Build history of the part. All positions in model axes, mm. Face numbers are marked on the shaded views. Round coordinates to 2 decimals unless told otherwise and drop trailing zeros. Loops run counter-clockwise (first coordinate to the right, second up) from the corner with the lowest first, then second, coordinate; pieces in that order, holes last. Notation, with made-up numbers: (12.25, 58.25) -> (61.25, 58.25) arc R21 ccw to (61.25, 78.25) -> close; hole circle Ø4 at (-2, 18.25). An arc over 180 degrees is marked (long way). Put each result on its own line as item: value. Start each with the question number.
Item 1: Drill centre lines: probe 1 along Y at (x, z) = (60, 26.3); probe 2 along X at (y, z) = (19.5, 25.75); probe 3 along X at (y, z) = (9.5, 23). Where is each one in solid material? Low to high. Write a range as [from, to].
Item 2: Cut at C-C, the plane x = 115. List the corners of the cut face in (y, z).
Item 3: Pull direction Y, two halves, no side cores. Call the marked faces 1, 2, 3 and 4: +Y half, -Y half, draft (parallel to the pull), parting line (faces both ways), or undercut.
Item 4: Cut at A-A, the plane y = 5. List the corners of the cut face in (x, z).
Item 5: Cut at D-D, the plane z = 28.5. Count the separate pieces of the cut face and the enclosed holes in it, plus the area to 3 significant figures.
Item 6: Flat gauge pin, fed straight in: pin 1 Ø0.8 at (x, z) = (61, 23.5) entering from +Y. Where does the tip first touch, or does it go through?
Item 7: Cut at B-B, the plane x = 5. List the corners of the cut face in (y, z).
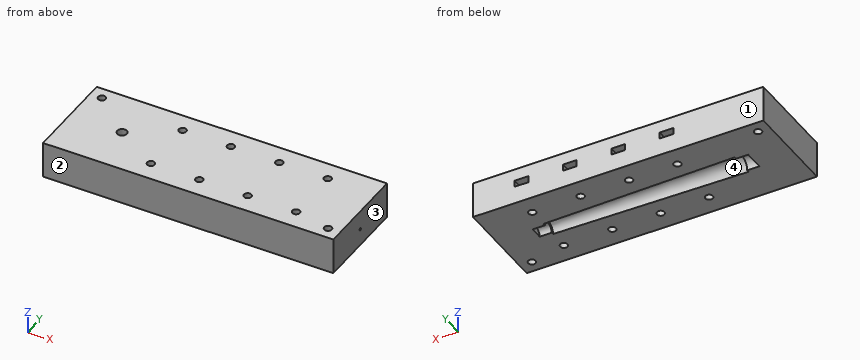
```python
from build123d import *

# Parameters (mm, degrees)
SKIZZE2_W                        = 120
SKIZZE2_H                        = 39.364160046
AUFSATZ_LINEAR_AUSTRAGEN1_DEPTH  = 30
SKIZZE24_R                       = 1.55
SCHNITT_LINEAR_AUSTRAGEN4_DEPTH  = 130.805766806
SKIZZE46_R                       = 2.85
SCHNITT_LINEAR_AUSTRAGEN15_DEPTH = 10
SCHNITT_LINEAR_START             = -5
SCHNITT_LINEAR_AUSTRAGEN25_DEPTH = 2.7
LINEARES_MUSTER1_COUNT           = 4
LINEARES_MUSTER1_PITCH           = 20
SPIEGELN2_COPY_1_SKETCH_R        = 2.85
SPIEGELN2_COPY_1_DEPTH           = 10
SPIEGELN2_COPY_2_SKETCH_R        = 2.85
SPIEGELN2_COPY_2_DEPTH           = 10
SPIEGELN2_COPY_3_SKETCH_R        = 2.85
SPIEGELN2_COPY_3_DEPTH           = 10
SPIEGELN2_START                  = -5
SPIEGELN2_COPY_4_DEPTH           = 2.7
SPIEGELN2_COPY_5_DEPTH           = 2.7
SPIEGELN2_COPY_6_DEPTH           = 2.7
SKIZZE51_R                       = 1.55
SCHNITT_LINEAR_AUSTRAGEN26_DEPTH = 130.805766806
SKIZZE75_R                       = 0.75
SCHNITT_LINEAR_AUSTRAGEN28_DEPTH = 12
SKIZZE76_R                       = 2
SCHNITT_LINEAR_AUSTRAGEN29_DEPTH = 6
SKIZZE80_R                       = 0.5
SCHNITT_LINEAR_AUSTRAGEN34_DEPTH = 21.05
SCHNITT_LINEAR_START_2           = -7.5
SKIZZE81_R                       = 0.5
SCHNITT_LINEAR_AUSTRAGEN36_DEPTH = 5
FASE1_SIZE                       = 1
ABSPALTEN3_OUTLINE_W             = 120
ABSPALTEN3_OUTLINE_H             = 39.364160046
ABSPALTEN3_OUTLINE_R             = 1.55
ABSPALTEN3_DEPTH                 = 15


# Read off the part's stored shape, not the designer's step: Abspalten3
with BuildPart() as part:
    # Skizze2 → Aufsatz-Linear austragen1 (new body)
    with BuildSketch(Plane.XY):
        with Locations((60, 19.682080023)):
            Rectangle(SKIZZE2_W, SKIZZE2_H)
    extrude(amount=AUFSATZ_LINEAR_AUSTRAGEN1_DEPTH)

    # Skizze24 → Schnitt-Linear austragen4 (cut, through all)
    with BuildSketch(Plane.XY.offset(30)):
        with Locations((40, 31.364160046)):
            Circle(SKIZZE24_R)
        with Locations((60, 31.364160046)):
            Circle(SKIZZE24_R)
        with Locations((80, 31.364160046)):
            Circle(SKIZZE24_R)
        with Locations((100, 31.364160046)):
            Circle(SKIZZE24_R)
    schnitt_linear_austragen4 = extrude(amount=-SCHNITT_LINEAR_AUSTRAGEN4_DEPTH, mode=Mode.SUBTRACT)

    # Skizze46 → Schnitt-Linear austragen15 (cut)
    with BuildSketch(Plane(origin=(0, 0, 0), x_dir=(-1, 0, 0), z_dir=(0, 0, -1))):
        with Locations((-100, 31.364160046)):
            Circle(SKIZZE46_R)
    schnitt_linear_austragen15 = extrude(amount=-SCHNITT_LINEAR_AUSTRAGEN15_DEPTH, mode=Mode.SUBTRACT)

    # Skizze50 → Schnitt-Linear austragen25 (cut)
    with BuildSketch(Plane.XY.offset(30).offset(SCHNITT_LINEAR_START)):
        Polygon((97.15, 33.009608314), (97.15, 39.364160046), (102.85, 39.364160046), (102.85, 33.009608314), (102.85, 29.718711779), (100, 28.073263512), (97.15, 29.718711779), align=None)
    schnitt_linear_austragen25 = extrude(amount=-SCHNITT_LINEAR_AUSTRAGEN25_DEPTH, mode=Mode.SUBTRACT)

    # Lineares Muster1: Schnitt-Linear austragen15, Schnitt-Linear austragen25 ×4
    with Locations(*[(-i * LINEARES_MUSTER1_PITCH, 0, 0) for i in range(1, LINEARES_MUSTER1_COUNT)]):
        add(schnitt_linear_austragen15, mode=Mode.SUBTRACT)
        add(schnitt_linear_austragen25, mode=Mode.SUBTRACT)

    # Spiegeln2: Schnitt-Linear austragen15, Schnitt-Linear austragen25 across plane
    add(schnitt_linear_austragen15.mirror(Plane.ZX.offset(19.764160046)), mode=Mode.SUBTRACT)
    add(schnitt_linear_austragen25.mirror(Plane.ZX.offset(19.764160046)), mode=Mode.SUBTRACT)

    # Spiegeln2 copy 1 sketch → Spiegeln2 copy 1 (cut)
    with BuildSketch(Plane(origin=(-20, 39.528320093, 0), x_dir=(-1, 0, 0), z_dir=(0, 0, -1))):
        with Locations((-100, -31.364160046)):
            Circle(SPIEGELN2_COPY_1_SKETCH_R)
    extrude(amount=-SPIEGELN2_COPY_1_DEPTH, mode=Mode.SUBTRACT)

    # Spiegeln2 copy 2 sketch → Spiegeln2 copy 2 (cut)
    with BuildSketch(Plane(origin=(-40, 39.528320093, 0), x_dir=(-1, 0, 0), z_dir=(0, 0, -1))):
        with Locations((-100, -31.364160046)):
            Circle(SPIEGELN2_COPY_2_SKETCH_R)
    extrude(amount=-SPIEGELN2_COPY_2_DEPTH, mode=Mode.SUBTRACT)

    # Spiegeln2 copy 3 sketch → Spiegeln2 copy 3 (cut)
    with BuildSketch(Plane(origin=(-60, 39.528320093, 0), x_dir=(-1, 0, 0), z_dir=(0, 0, -1))):
        with Locations((-100, -31.364160046)):
            Circle(SPIEGELN2_COPY_3_SKETCH_R)
    extrude(amount=-SPIEGELN2_COPY_3_DEPTH, mode=Mode.SUBTRACT)

    # Spiegeln2 copy 4 sketch → Spiegeln2 copy 4 (cut)
    with BuildSketch(Plane(origin=(-20, 39.528320093, 30), x_dir=(1, 0, 0), z_dir=(0, 0, 1)).offset(SPIEGELN2_START)):
        Polygon((97.15, -33.009608314), (97.15, -39.364160046), (102.85, -39.364160046), (102.85, -33.009608314), (102.85, -29.718711779), (100, -28.073263512), (97.15, -29.718711779), align=None)
    extrude(amount=-SPIEGELN2_COPY_4_DEPTH, mode=Mode.SUBTRACT)

    # Spiegeln2 copy 5 sketch → Spiegeln2 copy 5 (cut)
    with BuildSketch(Plane(origin=(-40, 39.528320093, 30), x_dir=(1, 0, 0), z_dir=(0, 0, 1)).offset(SPIEGELN2_START)):
        Polygon((97.15, -33.009608314), (97.15, -39.364160046), (102.85, -39.364160046), (102.85, -33.009608314), (102.85, -29.718711779), (100, -28.073263512), (97.15, -29.718711779), align=None)
    extrude(amount=-SPIEGELN2_COPY_5_DEPTH, mode=Mode.SUBTRACT)

    # Spiegeln2 copy 6 sketch → Spiegeln2 copy 6 (cut)
    with BuildSketch(Plane(origin=(-60, 39.528320093, 30), x_dir=(1, 0, 0), z_dir=(0, 0, 1)).offset(SPIEGELN2_START)):
        Polygon((97.15, -33.009608314), (97.15, -39.364160046), (102.85, -39.364160046), (102.85, -33.009608314), (102.85, -29.718711779), (100, -28.073263512), (97.15, -29.718711779), align=None)
    extrude(amount=-SPIEGELN2_COPY_6_DEPTH, mode=Mode.SUBTRACT)

    # Spiegeln3: Schnitt-Linear austragen4 across plane
    add(schnitt_linear_austragen4.mirror(Plane.ZX.offset(19.764160046)), mode=Mode.SUBTRACT)

    # Skizze51 → Schnitt-Linear austragen26 (cut, through all)
    with BuildSketch(Plane.XY.offset(30)):
        with Locations((5, 34.364160046)):
            Circle(SKIZZE51_R)
        with Locations((115, 5)):
            Circle(SKIZZE51_R)
    extrude(amount=-SCHNITT_LINEAR_AUSTRAGEN26_DEPTH, mode=Mode.SUBTRACT)

    # Skizze73 → Schnitt-Rotation5 (revolve, cut)
    with BuildSketch(Plane.XY.offset(15)):
        Polygon((15, 19.764160046), (15, 23.814160046), (20, 23.814160046), (20, 24.814160046), (100, 23.232080023), (100, 22.232080023), (105, 22.232080023), (105, 19.682080023), align=None)
    revolve(axis=Axis((105, 19.682080023, 15), (-0.9999995841280241, 0.0009119998787298228, 0)), mode=Mode.SUBTRACT)

    # Skizze75 → Schnitt-Linear austragen28 (cut)
    with BuildSketch(Plane.XY.offset(30)):
        with Locations((21.598259807, 19.682080023)):
            Circle(SKIZZE75_R)
    extrude(amount=-SCHNITT_LINEAR_AUSTRAGEN28_DEPTH, mode=Mode.SUBTRACT)

    # Skizze76 → Schnitt-Linear austragen29 (cut)
    with BuildSketch(Plane.XY.offset(30)):
        with Locations((21.598259807, 19.682080023)):
            Circle(SKIZZE76_R)
    extrude(amount=-SCHNITT_LINEAR_AUSTRAGEN29_DEPTH, mode=Mode.SUBTRACT)

    # Skizze80 → Schnitt-Linear austragen34 (cut)
    with BuildSketch(Plane(origin=(120, 0, 0), x_dir=(0, 0, -1), z_dir=(1, 0, 0))):
        with Locations((-22.000416524, 19.763714623)):
            Circle(SKIZZE80_R)
    schnitt_linear_austragen34 = extrude(amount=-SCHNITT_LINEAR_AUSTRAGEN34_DEPTH, mode=Mode.SUBTRACT)

    # Skizze81 → Schnitt-Linear austragen36 (cut)
    with BuildSketch(Plane.XY.offset(30).offset(SCHNITT_LINEAR_START_2)):
        with Locations(Location((99, 19.682080023, 0), (0, 0, 7.034090001))):
            Circle(SKIZZE81_R)
    schnitt_linear_austragen36 = extrude(amount=-SCHNITT_LINEAR_AUSTRAGEN36_DEPTH, mode=Mode.SUBTRACT)

    # Spiegeln4: Schnitt-Linear austragen34, Schnitt-Linear austragen36 across plane
    add(schnitt_linear_austragen34.mirror(Plane.XY.offset(15)), mode=Mode.SUBTRACT)
    add(schnitt_linear_austragen36.mirror(Plane.XY.offset(15)), mode=Mode.SUBTRACT)

    # Fase1
    fase1_edges = [part.edges().sort_by_distance(p)[0] for p in [
        (20.848259807, 19.682080023, 24),
    ]]
    chamfer(fase1_edges, length=FASE1_SIZE)

    # Abspalten3 outline → Abspalten3 (cut)
    with BuildSketch(Plane.XY):
        with Locations((60, 19.682080023)):
            Rectangle(ABSPALTEN3_OUTLINE_W, ABSPALTEN3_OUTLINE_H)
        with Locations((115, 5)):
            Circle(ABSPALTEN3_OUTLINE_R, mode=Mode.SUBTRACT)
        with Locations((5, 34.364160046)):
            Circle(ABSPALTEN3_OUTLINE_R, mode=Mode.SUBTRACT)
        with Locations((40, 8.164160046)):
            Circle(ABSPALTEN3_OUTLINE_R, mode=Mode.SUBTRACT)
        with Locations((60, 8.164160046)):
            Circle(ABSPALTEN3_OUTLINE_R, mode=Mode.SUBTRACT)
        with Locations((80, 8.164160046)):
            Circle(ABSPALTEN3_OUTLINE_R, mode=Mode.SUBTRACT)
        with Locations((100, 8.164160046)):
            Circle(ABSPALTEN3_OUTLINE_R, mode=Mode.SUBTRACT)
        with Locations((40, 31.364160046)):
            Circle(ABSPALTEN3_OUTLINE_R, mode=Mode.SUBTRACT)
        with Locations((60, 31.364160046)):
            Circle(ABSPALTEN3_OUTLINE_R, mode=Mode.SUBTRACT)
        with Locations((80, 31.364160046)):
            Circle(ABSPALTEN3_OUTLINE_R, mode=Mode.SUBTRACT)
        with Locations((100, 31.364160046)):
            Circle(ABSPALTEN3_OUTLINE_R, mode=Mode.SUBTRACT)
    extrude(amount=ABSPALTEN3_DEPTH, mode=Mode.SUBTRACT)


solid = part.part
```
Reply:
1. probe 1: y = [0, 6.61], [9.71, 29.81], [32.91, 39.36]
1. probe 2: x = [0, 19.61], [23.59, 120]
1. probe 3: x = [0, 37.15], [42.85, 57.15], [62.85, 77.15], [82.85, 97.15], [102.85, 120]
2. outline: (0, 15) -> (3.45, 15) -> (3.45, 30) -> (0, 30) -> close; (6.55, 15) -> (39.36, 15) -> (39.36, 30) -> (6.55, 30) -> close; hole circle Ø1 at (19.76, 22)
3. face 1: +Y half
3. face 2: -Y half
3. face 3: draft
3. face 4: undercut
4. outline: (0, 15) -> (113.45, 15) -> (113.45, 30) -> (0, 30) -> close; (116.55, 15) -> (120, 15) -> (120, 30) -> (116.55, 30) -> close; hole (37.15, 22.3) -> (42.85, 22.3) -> (42.85, 25) -> (37.15, 25) -> close; hole (57.15, 22.3) -> (62.85, 22.3) -> (62.85, 25) -> (57.15, 25) -> close; hole (77.15, 22.3) -> (82.85, 22.3) -> (82.85, 25) -> (77.15, 25) -> close; hole (97.15, 22.3) -> (102.85, 22.3) -> (102.85, 25) -> (97.15, 25) -> close
5. separate pieces: 1
5. enclosed holes: 11
5. area: 4,640 mm^2
6. pin 1: stops at y = 28.88
7. outline: (0, 15) -> (32.81, 15) -> (32.81, 30) -> (0, 30) -> close; (35.91, 15) -> (39.36, 15) -> (39.36, 30) -> (35.91, 30) -> close
